from build123d import *

# Parameters (mm, degrees)
CUT_EXTRUDE_1_DEPTH = 34.8
FILLET_1_R          = 5
CUT_EXTRUDE_2_REACH = 82.774
SKETCH_3_R          = 3.5


with BuildPart() as part:
    # Эскиз1 → Повернуть1 (revolve)
    with BuildSketch(Plane.XY, mode=Mode.PRIVATE) as revolve_1_sk:
        Polygon((0, 6.5), (15.2, 6.5), (15.2, 9.5), (4.7, 9.5), (4.7, 17.5), (35.2, 17.5), (35.2, 22.5), (55, 22.5), (55, 6.5), (70, 6.5), (70, 28.5), (34.8, 28.5), (34.8, 28), (0, 28), align=None)
    revolve(revolve_1_sk.sketch.rotate(Axis((-15.709814328, 0, 0), (1, 0, 0)), 90), axis=Axis((-15.709814328, 0, 0), (1, 0, 0)))

    # Эскиз2 → Вырез-Вытянуть1 (cut)
    with BuildSketch(Plane.ZY):
        with BuildLine():
            ThreePointArc((-7.5, 28.272115237), (0, 20.8), (7.5, 28.272115237))
            ThreePointArc((7.5, 28.272115237), (0, 29.25), (-7.5, 28.272115237))
        make_face()
        with BuildLine():
            ThreePointArc((20.734370014, 20.631248147), (18.013328399, 10.4), (28.234370014, 7.64086709))
            ThreePointArc((28.234370014, 7.64086709), (25.331243061, 14.625), (20.734370014, 20.631248147))
        make_face()
        with BuildLine():
            ThreePointArc((28.234370014, -7.64086709), (18.013328399, -10.4), (20.734370014, -20.631248147))
            ThreePointArc((20.734370014, -20.631248147), (25.331243061, -14.625), (28.234370014, -7.64086709))
        make_face()
        with BuildLine():
            ThreePointArc((7.5, -28.272115237), (0, -20.8), (-7.5, -28.272115237))
            ThreePointArc((-7.5, -28.272115237), (0, -29.25), (7.5, -28.272115237))
        make_face()
        with BuildLine():
            ThreePointArc((-20.734370014, -20.631248147), (-18.013328399, -10.4), (-28.234370014, -7.64086709))
            ThreePointArc((-28.234370014, -7.64086709), (-25.331243061, -14.625), (-20.734370014, -20.631248147))
        make_face()
        with BuildLine():
            ThreePointArc((-28.234370014, 7.64086709), (-18.013328399, 10.4), (-20.734370014, 20.631248147))
            ThreePointArc((-20.734370014, 20.631248147), (-25.331243061, 14.625), (-28.234370014, 7.64086709))
        make_face()
    extrude(amount=-CUT_EXTRUDE_1_DEPTH, mode=Mode.SUBTRACT)

    # Скругление1
    fillet_1_edges = [part.edges().sort_by_distance(p)[0] for p in [
        (34.8, 20.8, 0),
        (34.8, 10.4, 18.013328399),
        (34.8, -10.4, 18.013328399),
        (34.8, -20.8, 0),
        (34.8, -10.4, -18.013328399),
        (34.8, 10.4, -18.013328399),
    ]]
    fillet(fillet_1_edges, radius=FILLET_1_R)

    # Эскиз3 → Вырез-Вытянуть2 (cut, up to next)
    with BuildSketch(Plane(origin=(70, 0, 0), x_dir=(0, 0, -1), z_dir=(1, 0, 0)), mode=Mode.PRIVATE) as cut_extrude_2_sk1:
        with Locations((-17.5, 0)):
            Circle(SKETCH_3_R)
    cut_extrude_2_tool1 = extrude(cut_extrude_2_sk1.sketch, amount=-CUT_EXTRUDE_2_REACH, mode=Mode.PRIVATE) & part.part
    # Эскиз3 → Вырез-Вытянуть2 (cut, up to next)
    with BuildSketch(Plane(origin=(70, 0, 0), x_dir=(0, 0, -1), z_dir=(1, 0, 0)), mode=Mode.PRIVATE) as cut_extrude_2_sk2:
        with Locations((17.5, 0)):
            Circle(SKETCH_3_R)
    cut_extrude_2_tool2 = extrude(cut_extrude_2_sk2.sketch, amount=-CUT_EXTRUDE_2_REACH, mode=Mode.PRIVATE) & part.part
    add(cut_extrude_2_tool1.solids().sort_by_distance((70, 0, 17.5))[0], mode=Mode.SUBTRACT)
    add(cut_extrude_2_tool2.solids().sort_by_distance((70, 0, -17.5))[0], mode=Mode.SUBTRACT)


solid = part.part
For this review, take the finished solid that the model builds, in its own axes (mm). A direction names the side the tool comes from. Give positions to 0.01 mm unless a question says otherwise; leave off trailing zeros. Loops run counter-clockwise (first coordinate to the right, second up) from the corner with the lowest first, then second, coordinate; pieces in that order, holes last. Notation, with made-up numbers: M 68,-25.75 L 101,-25.75 A11 ccw 101,-20.75 Z; hole C 43.5,89.5 d11. An arc over 180 degrees is marked long. Answer as a JSON object with one key per item and string values. Group by question number.
Q1. For probe 1 along X at (y, z) = (-17.5, 10.5); probe 2 along X at (y, z) = (-13.5, 7.5); probe 3 along Y at (x, z) = (60.5, 0), list the stretches that pass through material, from the lowest coordinate up. Write a range as [from, to].
Q2. Add section A-A on x = 17. Give the boundary of the cut face in (y, z).
Q3. Add section C-C on x = 60.5. Give the boundary of the cut face in (y, z).
Q4. Mouldability with a two-part tool opening along Y and no side actions: class faces 1 (the cylindrical face through (17.16, -24.16, 14.15)), 2 (the cylindrical face through (14.69, -10.27, 18.09)), 3 (the cylindrical face through (17, 0, -28)) as +Y half, -Y half, draft (parallel to the pull), parting line (faces both ways), or undercut.
Q5. Tool access review of faces 4 (the cylindrical face through (62.6, 1.05, 14.16)), 5 (the cylindrical face through (17, 0, 28)), 6 (the cylindrical face through (17.16, 24.16, -14.15)): name each direction out of +Z, -Z, +X, -X, +Y, -Y from which nothing blocks a thin tool from reaching the whole face with its end or side.
Q6. Add section D-D on x = 48. Give the boundary of the cut face in (y, z), and give its area (3 significant figures).
Q7. Insertion check: P1, Ø1.5, axis at x = 27, z = 20.5, coming from the +Y side; P2, Ø1.5, axis at x = 57, z = 16.5, coming from the -Y side; P3, Ø1, axis at x = 27.5, z = 20.5, coming from the +Y side. Each pin has a flat end and moves straight along its axis. Give the tip position at first contact, or say it passes through.
Q8. Add section B-B on y = 0. Give the number of separate pieces and of enclosed holes in the cut face, and give its area (3 significant figures).
Checked values:
{
 "1": {"probe 1": "[0, 35.2], [55, 70]", "probe 2": "[0, 4.7], [55, 70]", "probe 3": "[-28.5, -6.5], [6.5, 28.5]"},
 "2": {"outline": "M -27.01,-7.39 A28 ccw -19.9,-19.7 A7.5 cw -7.11,-27.08 A28 ccw 7.11,-27.08 A7.5 cw 19.9,-19.7 A28 ccw 27.01,-7.39 A7.5 cw 27.01,7.39 A28 ccw 19.9,19.7 A7.5 cw 7.11,27.08 A28 ccw -7.11,27.08 A7.5 cw -19.9,19.7 A28 ccw -27.01,7.39 A7.5 cw Z; hole C 0,0 d35"},
 "3": {"outline": "C 0,0 d57; hole C 0,0 d13; hole C 0,-17.5 d7; hole C 0,17.5 d7"},
 "4": {"face 1": "-Y half", "face 2": "undercut", "face 3": "parting line"},
 "5": {"face 4": "+X", "face 5": "+Z, -X", "face 6": "-Z, -X, +Y"},
 "6": {"outline": "C 0,0 d57; hole C 0,0 d45", "area": "961 mm²"},
 "7": {"P1": "y = 8.35", "P2": "y = -23.75", "P3": "y = 8.16"},
 "8": {"separate pieces": "4", "enclosed holes": "0", "area": "1,590 mm²"}
}
